Can you work these out from the model? Positions are in its coordinate system, mm. Face numbers are marked on the shaded views. A direction names the side the tool comes from. Coordinates: 2 decimals unless noted, no trailing zeros. Order: outer loops, then holes, each group sorted by start corner. A loop starts at its lowest first (then second) coordinate and runs counter-clockwise, first axis right, second up. Notation, with made-up numbers: (47.25, 68) -> (87.25, 68) arc R13 cw to (87.25, 85) -> close; hole circle Ø3 at (64, 42). An arc over 180 degrees is marked (long way). Answer as a JSON object with one key per item and string values. Group by question number.
(1) I want a section at D-D, the plane z = 11.5. List the corners of the cut face in (x, y) for me, plus the area to 3 significant figures.
(2) I want a section at A-A, the plane y = 0. List the corners of the cut face in (x, z) for me, plus the area to 3 significant figures.
(3) I want a section at B-B, the plane x = 22.5. List the corners of the cut face in (y, z) for me, plus the area to 3 significant figures.
(4) For pin 1 (1.7 mm diameter, centred on x = 0, y = -45.5, fed in from +Z), with a flat end and sliding along its axis, tell me the tip position at first contact or that it passes through.
(5) I want a section at C-C, the plane z = 43. List the corners of the cut face in (x, y) for me.
(6) Which directions (+Z, -Z, +X, -X, +Y, -Y) give clear straight access to the entire face, cutting with the end or side of a thin tool? Please do the marked faces 5 and 6.
(7) I need wall thicknesses on line 1 (Z direction, x = 70, y = 0); line 2 (Y direction, x = -16.5, z = 29); line 3 (X direction, y = -41.5, z = 22.5). Which ranges of each line are inside material? Lowest first, please.
(8) If we mould it in two halves opening along X, with no side actions, what happens to the marked faces 1, 2, 3 and 4? For each: pulls with the +X half, pulls with the -X half, needs draft (parallel to the pull), parting line crosses it, or undercut.
from build123d import *

# Parameters (mm, degrees)
F0_W     = 143.8258737326
F0_H     = 97.4392816424
F0_W_2   = 133.3957463503
F0_H_2   = 85.9112516046
F1_DEPTH = 50.8
F2_W     = 51.9433170557
F2_H     = 17.0282212257
F3_DEPTH = 97.4402816424
F5_D     = 12.7


with BuildPart() as f1:
    # F0 (on Top) → F1 (new body)
    with BuildSketch(Plane.XY):
        Rectangle(F0_W, F0_H)
        Rectangle(F0_W_2, F0_H_2, mode=Mode.SUBTRACT)
    extrude(amount=F1_DEPTH)

    # F2 (on face) → F3 (cut, through all)
    with BuildSketch(Plane(origin=(0, 48.7196408212, 0), x_dir=(-1, 0, 0), z_dir=(0, 1, 0))):
        with Locations((0, 42.2858893871)):
            Rectangle(F2_W, F2_H)
    extrude(amount=-F3_DEPTH, mode=Mode.SUBTRACT)

    # F5 (through all)
    with Locations(Plane(origin=(-71.9129368663, 0, 0), x_dir=(0, -1, 0), z_dir=(-1, 0, 0))):
        with Locations((0, 25.1146312803)):
            Hole(F5_D / 2)


solid = f1.part
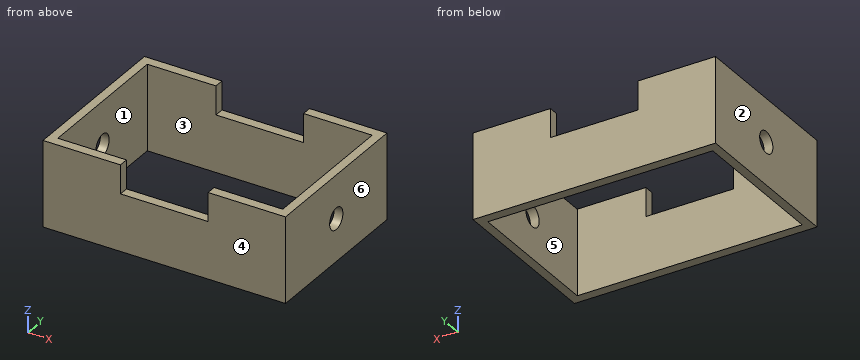
Computed values:
{
 "1": {"outline": "(-71.91, -48.72) -> (71.91, -48.72) -> (71.91, 48.72) -> (-71.91, 48.72) -> close; hole (-66.7, -42.96) -> (66.7, -42.96) -> (66.7, 42.96) -> (-66.7, 42.96) -> close", "area": "2,550 mm2"},
 "2": {"outline": "(-71.91, 0) -> (-66.7, 0) -> (-66.7, 18.76) -> (-71.91, 18.76) -> close; (-71.91, 31.46) -> (-66.7, 31.46) -> (-66.7, 50.8) -> (-71.91, 50.8) -> close; (66.7, 0) -> (71.91, 0) -> (71.91, 18.76) -> (66.7, 18.76) -> close; (66.7, 31.46) -> (71.91, 31.46) -> (71.91, 50.8) -> (66.7, 50.8) -> close", "area": "397 mm2"},
 "3": {"outline": "(-48.72, 0) -> (-42.96, 0) -> (-42.96, 33.77) -> (-48.72, 33.77) -> close; (42.96, 0) -> (48.72, 0) -> (48.72, 33.77) -> (42.96, 33.77) -> close", "area": "389 mm2"},
 "4": {"pin 1": "stops at z = 33.77"},
 "5": {"outline": "(-71.91, -48.72) -> (-25.97, -48.72) -> (-25.97, -42.96) -> (-66.7, -42.96) -> (-66.7, 42.96) -> (-25.97, 42.96) -> (-25.97, 48.72) -> (-71.91, 48.72) -> close; (25.97, -48.72) -> (71.91, -48.72) -> (71.91, 48.72) -> (25.97, 48.72) -> (25.97, 42.96) -> (66.7, 42.96) -> (66.7, -42.96) -> (25.97, -42.96) -> close"},
 "6": {"face 5": "+Z, -Z", "face 6": "+Z, -Z, +X, +Y, -Y"},
 "7": {"line 1": "z = 0 to 18.76, 31.46 to 50.8", "line 2": "y = -48.72 to -42.96, 42.96 to 48.72", "line 3": "x = -71.91 to -66.7, 66.7 to 71.91"},
 "8": {"face 1": "undercut", "face 2": "pulls with the -X half", "face 3": "undercut", "face 4": "needs draft"}
}
